from build123d import *

# Parameters (mm, degrees)
F0_W     = 60
F0_H     = 57
F1_DEPTH = 37
F3_DEPTH = 12
F4_W     = 20
F4_H     = 50
F5_DEPTH = 37.001


with BuildPart() as f1:
    # F0 (on Front) → F1 (new body)
    with BuildSketch(Plane.XZ):
        Rectangle(F0_W, F0_H)
    extrude(amount=F1_DEPTH)

    # F2 (on face) → F3 (cut)
    with BuildSketch(Plane.XY.offset(28.5)):
        Polygon((12, 0), (-12, 0), (-30, -18.5), (-30, -37), (30, -37), (30, -15.690912), align=None)
    extrude(amount=-F3_DEPTH, mode=Mode.SUBTRACT)

    # F4 (on face) → F5 (cut, through all)
    with BuildSketch(Plane.XZ.offset(37)):
        with Locations((0, -28.5)):
            Rectangle(F4_W, F4_H)
    extrude(amount=-F5_DEPTH, mode=Mode.SUBTRACT)


solid = f1.part
The model under review builds one solid part; all positions refer to its coordinate system, in mm. A direction names the side the tool comes from. Round coordinates to 2 decimals unless told otherwise and drop trailing zeros. Write each loop counter-clockwise with the first axis right and the second up, starting at its lowest first coordinate (ties: lowest second). Pieces come first, ordered by that corner, then holes. Notation, with made-up numbers: (77, -13.75) - (101, -13.75) arc R9 ccw to (101, -2.75) - close; hole circle Ø10 at (81, 1). An arc over 180 degrees is marked (long way). One line per item, written item: value. Start each with the question number.
1. To check wall thickness, follow L1, parallel to X at y = -27.5, z = -25; L2, parallel to Z at x = 11.5, y = -23.5; L3, parallel to Z at x = -6.5, y = -27. State the ranges of each line that lie inside material, in increasing order. Write a range as from..to.
2. Consider section B-B on z = -7.5. Write out the cut boundary in (x, y), and give its area (3 significant figures).
3. Consider section A-A on y = -29. Write out the cut boundary in (x, z).
4. The part is to be moulded in two halves that separate along X. For faces 4 (the face through (30, -18, 0)), 5 (the face through (-20, -18, -28.5)), 6 (the face through (0, -19, -3.5)), say which applies: released by +X, released by -X, zero draft, split by the parting line, or undercut.
5. Consider section D-D on z = 25.5. Write out the cut boundary in (x, y).
6. Consider section C-C on x = 17. Write out the cut boundary in (y, z), and give its area (3 significant figures).
7. Machinability: for faces 1 (the face through (-10, -19, -16)), 2 (the face through (-20.874, -9.121, 22.584)), 3 (the face through (-23, -7, 28.5)), which of the approach directions +Z, -Z, +X, -X, +Y, -Y give a long, thin tool a straight path to every point of the face, cutting with its end or side? Answer none if there is none.
8. Clearance check with flat-ended pins moving along their axes: P1, Ø6, axis at x = -18.5, y = -28, coming from the +Z side; P2, Ø4, axis at x = -11, z = 7, coming from the +Y side; P3, Ø6, axis at x = 1.5, y = -18.5, coming from the -Z side. State where each tip first meets the part, or that it passes through.
Checks:
1. L1: x = -30..-10, 10..30
1. L2: z = -28.5..16.5
1. L3: z = -3.5..16.5
2. outline: (-30, -37) - (-10, -37) - (-10, 0) - (-30, 0) - close; (10, -37) - (30, -37) - (30, 0) - (10, 0) - close
2. area: 1,480 mm^2
3. outline: (-30, -28.5) - (-10, -28.5) - (-10, -3.5) - (10, -3.5) - (10, -28.5) - (30, -28.5) - (30, 16.5) - (-30, 16.5) - close
4. face 4: released by +X
4. face 5: zero draft
4. face 6: undercut
5. outline: (-30, -18.5) - (-12, 0) - (-30, 0) - close; (12, 0) - (30, -15.69) - (30, 0) - close
6. outline: (-37, -28.5) - (0, -28.5) - (0, 28.5) - (-4.36, 28.5) - (-4.36, 16.5) - (-37, 16.5) - close
6. area: 1,720 mm^2
7. face 1: -Z, +Y, -Y
7. face 2: +Z, -Y
7. face 3: +Z, +X, -X, +Y, -Y
8. P1: stops at z = 16.5
8. P2: stops at y = 0
8. P3: stops at z = -3.5
